For this review, take the finished solid that the model builds, in its own axes (mm). A direction names the side the tool comes from. Give positions to 0.01 mm unless a question says otherwise; leave off trailing zeros. Loops run counter-clockwise (first coordinate to the right, second up) from the corner with the lowest first, then second, coordinate; pieces in that order, holes last.
Autodesk Inventor part; units mm, degrees
ref_plane "Work Plane2" through (0, 0, 250) normal (0, 0, 1) x (1, 0, 0)
ref_plane "YZ Plane" through (0, 0, 0) normal (1, 0, 0) x (0, 1, 0)
ref_plane "XZ Plane" through (0, 0, 0) normal (0, 1, 0) x (-1, 0, 0)
sketch "Sketch1" plane through (0, 0, 0) normal (0, 0, 1) x (1, 0, 0)
  circle A0 centre (0, 0) radius 35
  dimension "d0" = 70
extrude "Extrusion1" add sketch "Sketch1" along normal blind 500
sketch "Sketch2" plane through (0, 0, 500) normal (0, 0, 1) x (1, 0, 0)
  circle A0 centre (0, 0) radius 30
  dimension "d3" = 60
extrude "Extrusion2" cut sketch "Sketch2" against normal blind 500
sketch "Sketch3" plane through (0, 0, 500) normal (0, 0, 1) x (1, 0, 0)
  circle A0 centre (0, 0) radius 32.5
  dimension "d6" = 65
extrude "Extrusion3" cut sketch "Sketch3" against normal blind 10
ref_plane "Work Plane2" through (0, 0, 250) normal (0, 0, 1) x (1, 0, 0)
mirror "Mirror2" about plane through (0, 0, 250) normal (0, 0, 1) of "Extrusion3"
properties part number "project rolller 1 part2"
Q1. For pin 1 Ø4 at (y, z) = (-14, 133.5) entering from +X; pin 2 Ø2 at (x, y) = (15.5, -26) entering from +Z; pin 3 Ø1 at (x, z) = (-3.5, 340.5) entering from +Y, all flat-tipped, find the tip position at first contact; note any pin that passes through.
Answers:
pin 1: stops at x = 32.88
pin 2: stops at z = 490
pin 3: stops at y = 34.87
Q2. Mouldability with a two-part tool opening along X and no side actions: class faces 4 (the cylindrical face through (-28, 21, 246)), 5 (the flat face through (23.2, -23.2, 500)), 6 (the flat face through (-9, -29, 10)) as +X half, -X half, draft (parallel to the pull), parting line (faces both ways), or undercut.
Answers:
face 4: parting line
face 5: draft
face 6: undercut
Q3. Machinability: for faces 1 (the cylindrical face through (31, 9.76, 495.07)), 2 (the cylindrical face through (31, -9.76, 4.93)), 3 (the cylindrical face through (-29.97, 1.32, 253.36)), which of the approach directions +Z, -Z, +X, -X, +Y, -Y give a long, thin tool a straight path to every point of the face, cutting with its end or side? Answer none if there is none.
Answers:
face 1: +Z
face 2: -Z
face 3: +Z, -Z
Q4. Consider section C-C on z = 262.5. Give the boundary of the cut face in (x, y), plus the area to 3 significant figures.
Answers:
outline: circle Ø70 at (0, 0); hole circle Ø60 at (0, 0)
area: 1,020 mm2
Q5. For probe 1 along Y at (x, z) = (0, 268.5); probe 2 along Y at (x, z) = (0, 494); probe 3 along Z at (x, y) = (29, 10), list the stretches that pass through material, from the lowest coordinate up.
Answers:
probe 1: y = -35 to -30, 30 to 35
probe 2: y = -35 to -32.5, 32.5 to 35
probe 3: z = 10 to 490
Q6. Consider section A-A on x = 0. Give the boundary of the cut face in (y, z).
Answers:
outline: (-35, 0) - (-32.5, 0) - (-32.5, 10) - (-30, 10) - (-30, 490) - (-32.5, 490) - (-32.5, 500) - (-35, 500) - close; (30, 10) - (32.5, 10) - (32.5, 0) - (35, 0) - (35, 500) - (32.5, 500) - (32.5, 490) - (30, 490) - close
